Here's how the part is built. I have some questions about the finished solid (model axes, mm). Face numbers are marked on the shaded views. A direction names the side the tool comes from. Give positions to 0.01 mm unless a question says otherwise; leave off trailing zeros. Answer in a Markdown table with one row per item. Add a question column.
Item 1: We'd pull the mould along X, two halves only. Please class the marked faces 1, 2 and 3: released by +X, released by -X, zero draft, split by the parting line, or undercut.
Item 2: Which directions (+Z, -Z, +X, -X, +Y, -Y) give clear straight access to the entire face, cutting with the end or side of a thin tool? Please do the marked faces 4 and 5.
Item 3: If I drill on line 1 (Z direction, x = 0, y = 26); line 2 (X direction, y = 28.85, z = 0); line 3 (Y direction, x = 1.5, z = -0.75), over which ranges is the centre line in solid material (lowest first)?
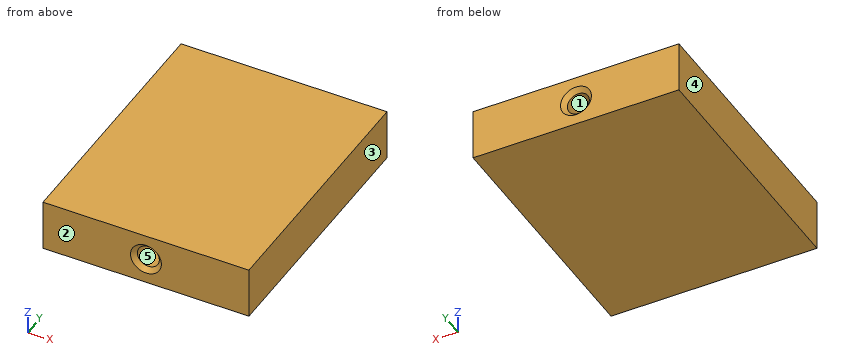
```python
from build123d import *

# Parameters (mm, degrees)
SKETCH1_W           = 50.8
SKETCH1_H           = 12.7
BOSS_EXTRUDE1_DEPTH = 31.75


with BuildPart() as part:
    # Sketch1 → Boss-Extrude1 (new body, symmetric)
    with BuildSketch(Plane(origin=(0, 0, 0), x_dir=(1, 0, 0), z_dir=(0, 1, 0))):
        Rectangle(SKETCH1_W, SKETCH1_H)
    extrude(amount=BOSS_EXTRUDE1_DEPTH, both=True)

    # Sketch3 → 1/4-28 Tapped Hole1 (revolve, cut)
    with BuildSketch(Plane(origin=(0, 31.75, 0), x_dir=(0, 0, 1), z_dir=(1, 0, 0))):
        Polygon((0, 0), (0, 7.975388061), (2.7051, 6.35), (2.7051, 1.1049), (3.81, 0), align=None)
    f_1_4_28_tapped_hole1 = revolve(axis=Axis((0, 38.1, 0), (0, -1, 0)), mode=Mode.SUBTRACT)

    # Mirror1: 1/4-28 Tapped Hole1 across plane
    add(f_1_4_28_tapped_hole1.mirror(Plane.ZX), mode=Mode.SUBTRACT)


solid = part.part
```
Recorded:
| question | item | result |
|---|---|---|
| 1 | face 1 | undercut |
| 1 | face 2 | zero draft |
| 1 | face 3 | released by +X |
| 2 | face 4 | +Z, -Z, -X, +Y, -Y |
| 2 | face 5 | -Y |
| 3 | line 1 | z = -6.35 to -2.71, 2.71 to 6.35 |
| 3 | line 2 | x = -25.4 to -2.71, 2.71 to 25.4 |
| 3 | line 3 | y = -24.78 to 24.78 |
